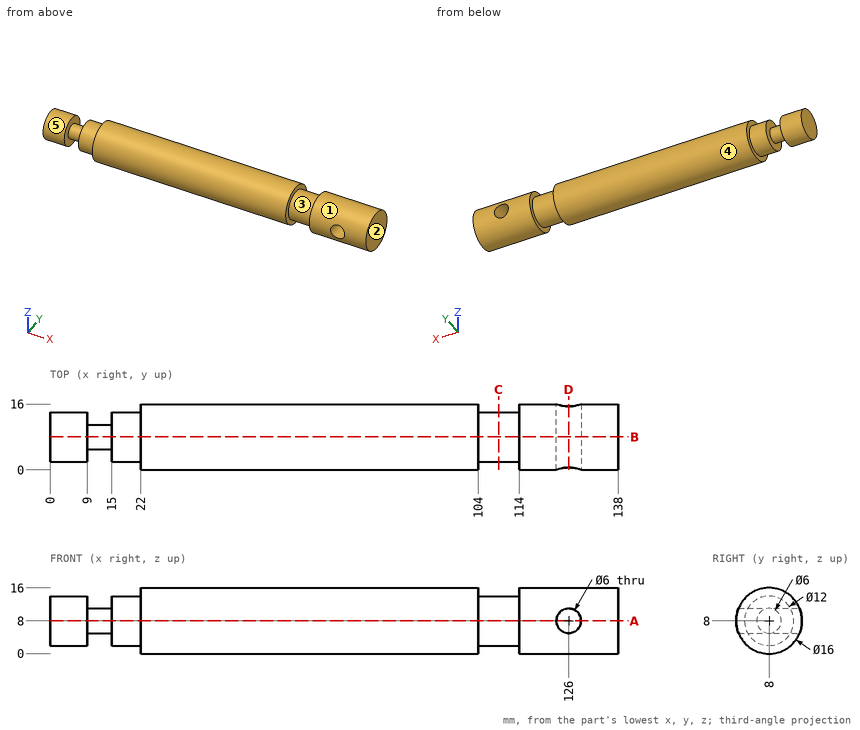
Verification items for this drawing (mm, ordinates from the low corner). A direction names the side the tool comes from. Give positions to 0.01 mm unless a question says otherwise; leave off trailing zeros. Loops run counter-clockwise (first coordinate to the right, second up) from the corner with the lowest first, then second, coordinate; pieces in that order, holes last. Notation, with made-up numbers: M 36,-23 L 41,-23 A19 cw 41,7 Z; hole C 40,-39 d1. An arc over 180 degrees is marked long. Return JSON: item names as keys, results as strings. Group by question number.
1. Mould release check, pull along X, two halves, no side actions. Record for the marked faces 1, 2 and 3: released by +X, released by -X, zero draft, split by the parting line, or undercut.
2. Go/stop test with flat-tipped pins: pin 1 (3 mm diameter, centred on x = 18, z = 9.5, fed in from +Y); pin 2 (3 mm diameter, centred on x = 98, y = 6, fed in from -Z); pin 3 (3 mm diameter, centred on x = 99, y = 10, fed in from +Z). Record where each tip stops, or that it passes through.
3. Tool access check on the marked faces 4 and 5. Record the directions out of +Z, -Z, +X, -X, +Y, -Y that give a thin tool (end or side, any length) a straight path to the whole face; none if there is none.
4. Cross-section at B-B on y = 8. Record the boundary of the cut face in (x, z).
5. Thickness scan on L1, parallel to X at y = 11.5, z = 1.75; L2, parallel to Z at x = 126, y = 8.75; L3, parallel to X at y = 5.25, z = 9. Record the ranges inside material, lowest first.
6. Cross-section at A-A on z = 8. Record the boundary of the cut face in (x, y).
7. Cross-section at D-D on x = 126. Record the boundary of the cut face in (y, z), plus the area to 3 significant figures.
8. Cross-section at C-C on x = 109. Record the boundary of the cut face in (y, z), plus the area to 3 significant figures.
Return value:
{
 "1": {"face 1": "zero draft", "face 2": "released by +X", "face 3": "undercut"},
 "2": {"pin 1": "y = 14", "pin 2": "z = 0.02", "pin 3": "z = 15.98"},
 "3": {"face 4": "+X, -X", "face 5": "-X"},
 "4": {"outline": "M 0,2 L 9,2 L 9,5 L 15,5 L 15,2 L 22,2 L 22,0 L 104,0 L 104,2 L 114,2 L 114,0 L 138,0 L 138,16 L 114,16 L 114,14 L 104,14 L 104,16 L 22,16 L 22,14 L 15,14 L 15,11 L 9,11 L 9,14 L 0,14 Z; hole C 126,8 d6"},
 "5": {"L1": "22 to 104, 114 to 138", "L2": "0.04 to 5, 11 to 15.96", "L3": "0 to 123.17, 128.83 to 138"},
 "6": {"outline": "M 0,2 L 9,2 L 9,5 L 15,5 L 15,2 L 22,2 L 22,0 L 104,0 L 104,2 L 114,2 L 114,0 L 123,0 L 123,16 L 114,16 L 114,14 L 104,14 L 104,16 L 22,16 L 22,14 L 15,14 L 15,11 L 9,11 L 9,14 L 0,14 Z; M 129,0 L 138,0 L 138,16 L 129,16 Z"},
 "7": {"outline": "M 0.58,5 A8 ccw 15.42,5 Z; M 0.58,11 L 15.42,11 A8 ccw Z", "area": "107 mm^2"},
 "8": {"outline": "C 8,8 d12", "area": "113 mm^2"}
}
